from build123d import *

# Parameters (mm, degrees)
SKETCH1_R           = 12.7
SKETCH1_R_2         = 4.7625
BOSS_EXTRUDE1_DEPTH = 609.6
SKETCH3_R           = 12.7
CUT_EXTRUDE1_DEPTH  = 6.35


with BuildPart() as part:
    # Sketch1 → Boss-Extrude1 (new body)
    with BuildSketch(Plane(origin=(0, 0, 0), x_dir=(1, 0, 0), z_dir=(0, 1, 0))):
        Circle(SKETCH1_R)
        Circle(SKETCH1_R_2, mode=Mode.SUBTRACT)
    extrude(amount=BOSS_EXTRUDE1_DEPTH)

    # Sketch3 → Cut-Extrude1 (cut)
    with BuildSketch(Plane.ZY.offset(12.7)):
        with Locations((0, 571.754)):
            Circle(SKETCH3_R)
    extrude(amount=-CUT_EXTRUDE1_DEPTH, mode=Mode.SUBTRACT)


solid = part.part
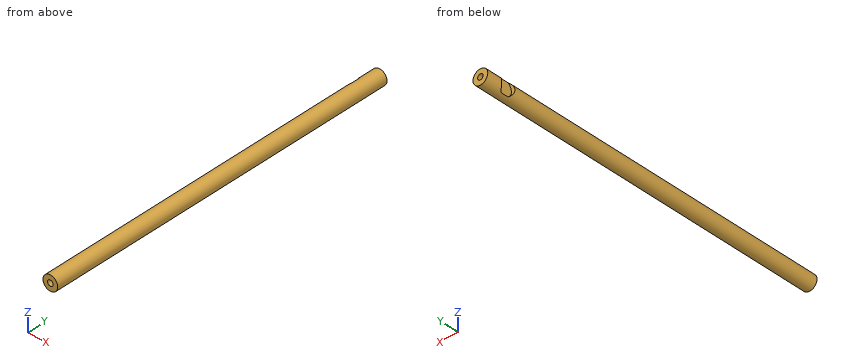
Source: CAD feature listing. Evaluate the final solid. Frame: model axes, mm. Give positions to 0.01 mm unless a question says otherwise; leave off trailing zeros. Order: outer loops, then holes, each group sorted by start corner. A loop starts at its lowest first (then second) coordinate and runs counter-clockwise, first axis right, second up. Notation, with made-up numbers: (73.25, 24.5) -> (120.25, 24.5) arc R19 ccw to (120.25, 51.5) -> close; hole circle Ø4 at (80.5, -22). An arc over 180 degrees is marked (long way). Write item = value, one per line.
Item 1: Section query B-B (x = 0). Output: boundary loops of the cut face in (y, z), then the cut area to 3 significant figures.
Check result:
outline = (0, -12.7) -> (609.6, -12.7) -> (609.6, -4.76) -> (0, -4.76) -> close; (0, 4.76) -> (609.6, 4.76) -> (609.6, 12.7) -> (0, 12.7) -> close
area = 9,680 mm²
Item 2: Section query C-C (y = 128.5). Output: boundary loops of the cut face in (x, z) (1 decimal), then the cut area to 3 significant figures.
Check result:
outline = circle Ø25.4 at (0, 0); hole circle Ø9.5 at (0, 0)
area = 435 mm²
Item 3: Ray query, probe 1 along Z at (x, y) = (0, 200); probe 2 along Z at (x, y) = (6.5, 435). Return the intervals inside material, ascending.
Check result:
probe_1 = -12.7 to -4.76, 4.76 to 12.7
probe_2 = -10.91 to 10.91
Item 4: Section query A-A (z = 0). Output: boundary loops of the cut face in (x, y), then the cut area to 3 significant figures.
Check result:
outline = (-12.7, 0) -> (-4.76, 0) -> (-4.76, 609.6) -> (-12.7, 609.6) -> (-12.7, 584.45) -> (-6.35, 584.45) -> (-6.35, 559.05) -> (-12.7, 559.05) -> close; (4.76, 0) -> (12.7, 0) -> (12.7, 609.6) -> (4.76, 609.6) -> close
area = 9,520 mm²
Item 5: Contact query for flat-ended pins moving along their axis: pin 1 (3 mm diameter, centred on x = -9, y = 291, fed in from +Z); pin 2 (2 mm diameter, centred on x = -8, y = 536.5, fed in from -Z); pin 3 (5 mm diameter, centred on y = 283, z = 9.5, fed in from +X). Output: stop coordinate, or through.
Check result:
pin_1 = 10.25
pin_2 = -10.6
pin_3 = 10.6
